Source: CAD feature listing. Evaluate the final solid. Frame: model axes, mm. Face numbers are marked on the shaded views. A direction names the side the tool comes from. Give positions to 0.01 mm unless a question says otherwise; leave off trailing zeros. Order: outer loops, then holes, each group sorted by start corner. A loop starts at its lowest first (then second) coordinate and runs counter-clockwise, first axis right, second up. Notation, with made-up numbers: (-38.5, 34) -> (-32.5, 34) arc R29 ccw to (-32.5, 68) -> close; hole circle Ø5 at (54.5, -22). An arc over 180 degrees is marked (long way). Answer in a Markdown table with one row per item.
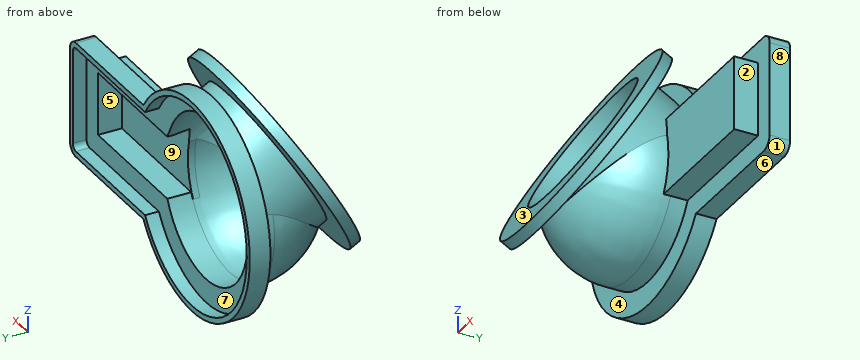
```python
from build123d import *

# Parameters (mm, degrees)
BOSS_EXTRUDE1_DEPTH     = 3.175
EXTRUDE_THIN1_START     = 7.874
EXTRUDE_THIN1_DEPTH     = 7.874
BOSS_EXTRUDE2_DEPTH     = 3.175
EXTRUDE_THIN2_REACH     = 134.494
SKETCH7_R               = 36.861935
SKETCH7_R_2             = 34.321935
CUT_EXTRUDE1_DEPTH      = 44.45
CUT_EXTRUDE1_DEPTH_BACK = 13.335
SKETCH8_R               = 34.321935
SKETCH10_R              = 50.8
SKETCH10_R_2            = 34.321935
BOSS_EXTRUDE3_DEPTH     = 5.08
FILLET1_START           = -1
FILLET1_DEPTH           = 5
BOSS_EXTRUDE4_START     = -3.175
BOSS_EXTRUDE4_DEPTH     = 9.525


with BuildPart() as part:
    # Sketch1 → Boss-Extrude1 (new body)
    with BuildSketch(Plane(origin=(0, 0, 0), x_dir=(1, 0, 0), z_dir=(0, 1, 0))):
        with BuildLine():
            Line((39.687895, -24.196019), (100.838, -24.196019))
            Line((100.838, -24.196019), (100.838, 24.196019))
            Line((100.838, 24.196019), (39.687895, 24.196019))
            ThreePointArc((39.687895, 24.196019), (-46.482, 0), (39.687895, -24.196019))
        make_face()
        with BuildLine():
            Line((32.449732, -14.544019), (91.186, -14.544019))
            Line((91.186, -14.544019), (91.186, 14.544019))
            Line((91.186, 14.544019), (32.449732, 14.544019))
            ThreePointArc((32.449732, 14.544019), (-35.56, 0), (32.449732, -14.544019))
        make_face(mode=Mode.SUBTRACT)
    extrude(amount=BOSS_EXTRUDE1_DEPTH)

    # Sketch4 → Extrude-Thin1 (add)
    with BuildSketch(Plane.XZ.offset(EXTRUDE_THIN1_START)):
        with BuildLine():
            Line((34.055048, 17.084019), (93.726, 17.084019))
            Line((93.726, 17.084019), (93.726, -17.084019))
            Line((93.726, -17.084019), (34.055048, -17.084019))
            ThreePointArc((34.055048, -17.084019), (-38.1, 0), (34.055048, 17.084019))
        make_face()
        with BuildLine():
            Line((32.449732, 14.544019), (91.186, 14.544019))
            Line((91.186, 14.544019), (91.186, -14.544019))
            Line((91.186, -14.544019), (32.449732, -14.544019))
            ThreePointArc((32.449732, -14.544019), (-35.56, 0), (32.449732, 14.544019))
        make_face(mode=Mode.SUBTRACT)
    extrude(amount=-EXTRUDE_THIN1_DEPTH)

    # Sketch5 → Revolve1 (revolve)
    with BuildSketch(Plane.XY):
        with BuildLine():
            Line((0, -43.434), (0, -45.974))
            ThreePointArc((0, -45.974), (-26.940768, -34.814768), (-38.1, -7.874))
            Line((-38.1, -7.874), (-35.56, -7.874))
            ThreePointArc((-35.56, -7.874), (-25.144717, -33.018717), (0, -43.434))
        make_face()
    revolve(axis=Axis((0, -50.818528, 0), (0, 1, 0)))

    # Sketch6 → Boss-Extrude2 (add)
    with BuildSketch(Plane.XZ.offset(7.874)):
        with BuildLine():
            Line((30.889366, -17.084019), (93.726, -17.084019))
            Line((93.726, -17.084019), (93.726, 17.084019))
            Line((93.726, 17.084019), (30.889366, 17.084019))
            ThreePointArc((30.889366, 17.084019), (35.298961, 0), (30.889366, -17.084019))
        make_face()
    extrude(amount=BOSS_EXTRUDE2_DEPTH)

    # Sketch7 → Extrude-Thin2 (add, up to next)
    with BuildSketch(Plane(origin=(0, -20.306958, 35.540261), x_dir=(1, 0, 0), z_dir=(0, 0.8661855860486005, -0.49972245348957706)), mode=Mode.PRIVATE) as extrude_thin2_sk1:
        with Locations((0, 19.05)):
            Circle(SKETCH7_R)
        with Locations((0, 19.05)):
            Circle(SKETCH7_R_2, mode=Mode.SUBTRACT)
    extrude_thin2_tool1 = extrude(extrude_thin2_sk1.sketch, amount=EXTRUDE_THIN2_REACH, mode=Mode.PRIVATE) - part.part
    add(extrude_thin2_tool1.solids().sort_by_distance((-35.819322, -29.826671, 19.039425))[0])

    # Sketch8 → Cut-Extrude1 (cut, two sides: drawn at the far end of the back side and taken through both)
    with BuildSketch(Plane(origin=(0, -20.306958, 35.540261), x_dir=(1, 0, 0), z_dir=(0, 0.8661855860486005, -0.49972245348957706)).offset(-CUT_EXTRUDE1_DEPTH_BACK)):
        with Locations(Location((0, 19.05, 0), (0, 0, 359.940086))):
            Circle(SKETCH8_R)
    extrude(amount=CUT_EXTRUDE1_DEPTH + CUT_EXTRUDE1_DEPTH_BACK, mode=Mode.SUBTRACT)

    # Sketch10 → Boss-Extrude3 (add)
    with BuildSketch(Plane(origin=(0, -30.61954, 17.665119), x_dir=(1, 0, 0), z_dir=(0, -0.8661855860486006, 0.49972245348957695))):
        with Locations(Location((0, 0, 0), (0, 0, 270))):
            Circle(SKETCH10_R)
        with Locations(Location((0, 1.586619, 0), (0, 0, 0.059914))):
            Circle(SKETCH10_R_2, mode=Mode.SUBTRACT)
    extrude(amount=-BOSS_EXTRUDE3_DEPTH)

    # Fillet1: read off the stored shape, not the designer's step
    # Fillet1 outline → Fillet1 (cut)
    with BuildSketch(Plane(origin=(0, 0, 0), x_dir=(1, 0, 0), z_dir=(0, 1, 0)).offset(FILLET1_START)):
        with BuildLine():
            Line((100.838, -24.196019), (100.838, -21.656019))
            ThreePointArc((100.838, -21.656019), (100.094051, -23.45207), (98.298, -24.196019))
            Line((98.298, -24.196019), (100.838, -24.196019))
        make_face()
        with BuildLine():
            ThreePointArc((98.298, 24.196019), (100.094051, 23.45207), (100.838, 21.656019))
            Line((100.838, 21.656019), (100.838, 24.196019))
            Line((100.838, 24.196019), (98.298, 24.196019))
        make_face()
    extrude(amount=FILLET1_DEPTH, mode=Mode.SUBTRACT)

    # Boss-Extrude4: read off the stored shape, not the designer's step
    # Boss-Extrude4 outline → Boss-Extrude4 (add)
    with BuildSketch(Plane(origin=(0, 3.175, 0), x_dir=(1, 0, 0), z_dir=(0, 1, 0)).offset(BOSS_EXTRUDE4_START)):
        with BuildLine():
            ThreePointArc((41.089436, 26.736019), (-49.022, 0), (41.089436, -26.736019))
            Line((41.089436, -26.736019), (98.298, -26.736019))
            ThreePointArc((98.298, -26.736019), (101.890102, -25.248122), (103.378, -21.656019))
            Line((103.378, -21.656019), (103.378, 21.656019))
            ThreePointArc((103.378, 21.656019), (101.890102, 25.248122), (98.298, 26.736019))
            Line((98.298, 26.736019), (41.089436, 26.736019))
        make_face()
        with BuildLine():
            Line((98.298, -24.196019), (39.687895, -24.196019))
            ThreePointArc((39.687895, -24.196019), (-46.482, 0), (39.687895, 24.196019))
            Line((39.687895, 24.196019), (98.298, 24.196019))
            ThreePointArc((98.298, 24.196019), (100.094051, 23.45207), (100.838, 21.656019))
            Line((100.838, 21.656019), (100.838, -21.656019))
            ThreePointArc((100.838, -21.656019), (100.094051, -23.45207), (98.298, -24.196019))
        make_face(mode=Mode.SUBTRACT)
    extrude(amount=BOSS_EXTRUDE4_DEPTH)


solid = part.part
```
(1) Section query A-A (x = 69). Return the cut outline in (y, z) (3 decimals), plus the area to 3 significant figures.
A:
| item | result |
|---|---|
| outline | (-11.049, -17.084) -> (0, -17.084) -> (0, -26.736) -> (9.525, -26.736) -> (9.525, -24.196) -> (3.175, -24.196) -> (3.175, -14.544) -> (-7.874, -14.544) -> (-7.874, 14.544) -> (3.175, 14.544) -> (3.175, 24.196) -> (9.525, 24.196) -> (9.525, 26.736) -> (0, 26.736) -> (0, 17.084) -> (-11.049, 17.084) -> close |
| area | 258 mm^2 |
(2) Access query for the marked faces 1, 2, 3, 4 and 5. Directions: +Z, -Z, +X, -X, +Y, -Y. A direction counts if a zero-diameter tool reaches every point of the face in a straight line with its end or side. Return the directions, or none.
A:
| item | result |
|---|---|
| face 1 | -Z, +X, +Y, -Y |
| face 2 | +Z, -Z, +X, -Y |
| face 3 | +Z, +X, -X, -Y |
| face 4 | none |
| face 5 | +Y |
(3) Pull-direction query (Z, two-part tool) for the marked faces 6, 7, 8 and 9; classes: +Z half, -Z half, draft (parallel to the pull), parting line (faces both ways), or undercut.
A:
| item | result |
|---|---|
| face 6 | -Z half |
| face 7 | undercut |
| face 8 | draft |
| face 9 | undercut |
(4) Ray query, probe 1 along Z at (x, y) = (24.5, -9); probe 2 along Z at (x, y) = (60.5, -4.5); probe 3 along Z at (x, y) = (0, 5). Return the intervals inside material, ascending.
A:
| item | result |
|---|---|
| probe 1 | z = -29.16 to -25.75, 34.77 to 38.82, 44.97 to 55.14 |
| probe 2 | z = -17.08 to -14.54, 14.54 to 17.08 |
| probe 3 | z = -49.02 to -46.48, 46.48 to 49.02 |
(5) First-contact query: pin 1 Ø7.5 at (x, y) = (62.5, 5) entering from +Z; pin 2 Ø12 at (x, y) = (62.5, -4.5) entering from -Z; pin 3 Ø10 at (x, y) = (73, -10) entering from +Z; pin 4 Ø12 at (x, z) = (68, -37) entering from -Y. Flat tips, straight axial feed; report the tip coordinate or a pass-through.
A:
| item | result |
|---|---|
| pin 1 | stops at z = 26.74 |
| pin 2 | stops at z = -26.74 |
| pin 3 | stops at z = 17.08 |
| pin 4 | passes through |
